from build123d import *

# Parameters (mm, degrees)
BOSS_EXTRUDE1_DEPTH = 3.96875
FILLET1_R           = 0.254
SHELL2_T            = -0.79375
SKETCH2_R           = 2.38125
BOSS_EXTRUDE2_DEPTH = 5.55625
SKETCH4_R           = 1.5875
CUT_EXTRUDE1_DEPTH  = 1.905
SKETCH5_R           = 1.5875
CUT_EXTRUDE2_DEPTH  = 1.905


with BuildPart() as part:
    # Sketch1 → Boss-Extrude1 (new, symmetric)
    with BuildSketch(Plane.XY):
        Polygon((0, 0), (15.08125, 0), (15.08125, 0.79375), (13.096875, 12.7), (1.984375, 12.7), (0, 0.79375), align=None)
    extrude(amount=BOSS_EXTRUDE1_DEPTH, both=True)

    # Fillet1
    fillet1_edges = [part.edges().sort_by_distance(p)[0] for p in [
        (1.984375, 12.7, 0),
        (13.096875, 12.7, 0),
        (15.08125, 0.396875, 3.96875),
        (14.0890625, 6.746875, 3.96875),
        (7.540625, 12.7, 3.96875),
        (0.9921875, 6.746875, 3.96875),
        (0, 0.396875, 3.96875),
        (0.9921875, 6.746875, -3.96875),
        (7.540625, 12.7, -3.96875),
        (14.0890625, 6.746875, -3.96875),
        (15.08125, 0.396875, -3.96875),
        (0, 0.396875, -3.96875),
    ]]
    fillet(fillet1_edges, radius=FILLET1_R)

    # Shell2
    shell2_openings = [part.faces().sort_by_distance(p)[0] for p in [
        (7.540625, 0, 0),
    ]]
    offset(amount=SHELL2_T, openings=shell2_openings, kind=Kind.INTERSECTION)

    # Sketch2 → Boss-Extrude2 (add)
    with BuildSketch(Plane(origin=(0, 12.7, 0), x_dir=(1, 0, 0), z_dir=(0, 1, 0))):
        with Locations((7.540625, 0)):
            Circle(SKETCH2_R)
    extrude(amount=BOSS_EXTRUDE2_DEPTH)

    # Sketch4 → Cut-Extrude1 (cut)
    with BuildSketch(Plane(origin=(14.802364865, 2.467060811, 0), x_dir=(0, 0, -1), z_dir=(0.9863939238321437, 0.16439898730535743, 0))):
        with Locations(Location((0, 7.045657773, 0), (0, 0, 90))):
            Circle(SKETCH4_R)
    extrude(amount=-CUT_EXTRUDE1_DEPTH, mode=Mode.SUBTRACT)

    # Sketch5 → Cut-Extrude2 (cut)
    with BuildSketch(Plane(origin=(-0.128716216, 0.021452703, 0), x_dir=(0, 0, 1), z_dir=(-0.9863939238321439, 0.16439898730535724, 0))):
        with Locations(Location((0, 9.525, 0), (0, 0, 270))):
            Circle(SKETCH5_R)
    extrude(amount=-CUT_EXTRUDE2_DEPTH, mode=Mode.SUBTRACT)


solid = part.part
The listing builds one solid part. Answer for the finished solid, in the listing's coordinates (mm). A direction names the side the tool comes from. Coordinates: 2 decimals unless noted, no trailing zeros. Write each loop counter-clockwise with the first axis right and the second up, starting at its lowest first coordinate (ties: lowest second). Pieces come first, ordered by that corner, then holes. Notation, with made-up numbers: (-32, -8.75) - (24, -8.75) arc R25 cw to (24, 6.25) - close; hole circle Ø11 at (18, 56). An arc over 180 degrees is marked (long way). Return JSON: item names as keys, results as strings.
1. For a pull along Z with two mould halves and no side action, classify faces 4 (the face through (14.12, 6.56, 0.05)), 5 (the face through (13.37, 6.24, 0.04)), 6 (the face through (7, 6, -3.969)), 7 (the face through (1.6, 7.9, -0.6)) as +Z half, -Z half, draft (parallel to the pull), parting line (faces both ways), or undercut.
Final values:
{"face 4": "draft", "face 5": "undercut", "face 6": "-Z half", "face 7": "undercut"}
2. Consider line 1 along Z through (x, y) = (3.75, 7.5) (3 decimals); line 2 along Y through (x, z) = (3.5, 2.75); line 3 along Y through (x, z) = (7.75, -0.25). Determine where each line is inside the solid, lowest interval first.
Final values:
{"line 1": "-3.969 to -3.175, 3.175 to 3.969", "line 2": "11.91 to 12.7", "line 3": "11.91 to 18.26"}
3. This flat-tipped pin is pushed along its axis until it touches: pin 1 Ø1.9 at (x, z) = (5.5, 0) entering from -Y. Where does it stop, or does it pass through?
Final values:
{"pin 1": "y = 11.91"}
4. The part is cut by section A-A on z = 0. Determine the outline of the cut face in (x, y), then the cut area to 3 significant figures.
Final values:
{"outline": "(0, 0) - (0.79, 0) - (0.79, 0.73) - (1.96, 7.72) - (1.18, 7.85) - (0, 0.79) - close; (1.7, 10.98) - (2.48, 10.85) - (2.66, 11.91) - (12.42, 11.91) - (12.6, 10.85) - (13.38, 10.98) - (13.13, 12.49) arc R0.25 ccw to (12.88, 12.7) - (9.92, 12.7) - (9.92, 18.26) - (5.16, 18.26) - (5.16, 12.7) - (2.2, 12.7) arc R0.25 ccw to (1.95, 12.49) - close; (13.12, 7.72) - (14.29, 0.73) - (14.29, 0) - (15.08, 0) - (15.08, 0.79) - (13.91, 7.85) - close", "area": "49.5 mm^2"}
5. The part is cut by section D-D on y = 15.25. Determine the outline of the cut face in (x, z), then the cut area to 3 significant figures.
Final values:
{"outline": "circle Ø4.76 at (7.54, 0)", "area": "17.8 mm^2"}
6. Which of the six approach directions +Z, -Z, +X, -X, +Y, -Y give full straight-line access (tool end or side, diameter ignored) to faces 1 (the face through (14.022, 6.711, 3.892)), 2 (the face through (7, 6, -3.175)), 3 (the face through (8, 12.7, 3))?
Final values:
{"face 1": "+Z, +X, +Y", "face 2": "-Y", "face 3": "+Y"}
7. The part is cut by section B-B on x = 4.5. Determine the outline of the cut face in (y, z) (3 decimals), then the cut area to 3 significant figures.
Final values:
{"outline": "(0, -3.969) - (12.446, -3.969) arc R0.254 ccw to (12.7, -3.715) - (12.7, 3.715) arc R0.254 ccw to (12.446, 3.969) - (0, 3.969) - (0, 3.175) - (11.906, 3.175) - (11.906, -3.175) - (0, -3.175) - close", "area": "25.2 mm^2"}
8. The part is cut by section C-C on z = -2.75. Determine the outline of the cut face in (x, y), then the cut area to 3 significant figures.
Final values:
{"outline": "(0, 0) - (0.79, 0) - (0.79, 0.73) - (2.66, 11.91) - (12.42, 11.91) - (14.29, 0.73) - (14.29, 0) - (15.08, 0) - (15.08, 0.79) - (13.13, 12.49) arc R0.25 ccw to (12.88, 12.7) - (2.2, 12.7) arc R0.25 ccw to (1.95, 12.49) - (0, 0.79) - close", "area": "28.1 mm^2"}
